The model under review builds one solid part; all positions refer to its coordinate system, in mm. A direction names the side the tool comes from. Give positions to 0.01 mm unless a question says otherwise; leave off trailing zeros. Order: outer loops, then holes, each group sorted by start corner. A loop starts at its lowest first (then second) coordinate and runs counter-clockwise, first axis right, second up.
```python
from build123d import *

# Parameters (mm, degrees)
F1_DEPTH = 19.05
F2_R     = 28.575
F3_DEPTH = 19.051
F4_R     = 12.7
F5_DEPTH = 15.24


with BuildPart() as f1:
    # F0 (on Top) → F1 (new body)
    with BuildSketch(Plane.XY):
        with BuildLine():
            ThreePointArc((133.35, 127), (125.910512, 144.960512), (107.95, 152.4))
            Line((107.95, 152.4), (0, 152.4))
            Line((0, 152.4), (0, -152.4))
            Line((0, -152.4), (107.95, -152.4))
            ThreePointArc((107.95, -152.4), (125.910512, -144.960512), (133.35, -127))
            Line((133.35, -127), (133.35, 127))
        make_face()
        with BuildLine():
            Line((0, -152.4), (0, 152.4))
            Line((0, 152.4), (-107.95, 152.4))
            ThreePointArc((-107.95, 152.4), (-125.910512, 144.960512), (-133.35, 127))
            Line((-133.35, 127), (-133.35, -127))
            ThreePointArc((-133.35, -127), (-125.910512, -144.960512), (-107.95, -152.4))
            Line((-107.95, -152.4), (0, -152.4))
        make_face()
    extrude(amount=F1_DEPTH)

    # F2 (on face) → F3 (cut, through all)
    with BuildSketch(Plane.XY.offset(19.05)):
        with Locations((-55.88, 100.965)):
            Circle(F2_R)
        with Locations((-55.88, 33.655)):
            Circle(F2_R)
        with Locations((-55.88, -33.655)):
            Circle(F2_R)
        with Locations((-55.88, -100.965)):
            Circle(F2_R)
        with Locations((55.88, -100.965)):
            Circle(F2_R)
        with Locations((55.88, -33.655)):
            Circle(F2_R)
        with Locations((55.88, 33.655)):
            Circle(F2_R)
        with Locations((55.88, 100.965)):
            Circle(F2_R)
    extrude(amount=-F3_DEPTH, mode=Mode.SUBTRACT)

    # F4 (on face) → F5 (cut)
    with BuildSketch(Plane.XY.offset(19.05)):
        with Locations((0, 96.52)):
            Circle(F4_R)
        with Locations((0, -96.52)):
            Circle(F4_R)
    extrude(amount=-F5_DEPTH, mode=Mode.SUBTRACT)


solid = f1.part
```
Item 1: Take a section at B-B (y = -96.52). Give the boundary of the cut face in (x, z), and give its area (3 significant figures).
Values found:
outline: (-133.35, 0) - (-84.11, 0) - (-84.11, 19.05) - (-133.35, 19.05) - close; (-27.65, 0) - (27.65, 0) - (27.65, 19.05) - (12.7, 19.05) - (12.7, 3.81) - (-12.7, 3.81) - (-12.7, 19.05) - (-27.65, 19.05) - close; (84.11, 0) - (133.35, 0) - (133.35, 19.05) - (84.11, 19.05) - close
area: 2,540 mm2
Item 2: Draft analysis for pull direction X (two halves, no side actions). For faces 1 (the flat face through (-2, 2, 19.05)), 2 (the cylindrical face through (125.71, -145.16, 9.39)), 3 (the cylindrical face through (-62.07, 73.07, 9.66)), state which applies: released by +X, released by -X, zero draft, split by the parting line, or undercut.
Values found:
face 1: zero draft
face 2: released by +X
face 3: undercut
Item 3: Clearance check with a flat-ended pin moving along its axis: pin 1 Ø7.5 at (x, y) = (6, 96) entering from +Z. State where the tip first meets the part, or that it passes through.
Values found:
pin 1: stops at z = 3.81
Item 4: Take a section at C-C (z = 7.5). Give the number of separate pieces and of enclosed holes in the cut face, and give its area (3 significant figures).
Values found:
separate pieces: 1
enclosed holes: 10
area: 59,200 mm2
Item 5: For faces 4 (the flat face through (0, -96, 3.81)), 5 (the cylindrical face through (-126.11, -144.76, 9.39)), list the 3-axis set-ups (+Z, -Z, +X, -X, +Y, -Y) from which the entire face can be reached by the end or side of a thin tool; tool diameter is ignored.
Values found:
face 4: +Z
face 5: +Z, -Z, -X, -Y
Item 6: For line 1 (X direction, y = -33, z = 3.75); line 2 (Y direction, x = -55.88, z = 5.25); line 3 (Y direction, x = 58, z = 11.5), list the stretches that pass through material, from the lowest coordinate up.
Values found:
line 1: x = -133.35 to -84.45, -27.31 to 27.31, 84.45 to 133.35
line 2: y = -152.4 to -129.54, -72.39 to -62.23, -5.08 to 5.08, 62.23 to 72.39, 129.54 to 152.4
line 3: y = -152.4 to -129.46, -72.47 to -62.15, -5.16 to 5.16, 62.15 to 72.47, 129.46 to 152.4
Item 7: Take a section at D-D (x = 0). Give the boundary of the cut face in (y, z).
Values found:
outline: (-152.4, 0) - (152.4, 0) - (152.4, 19.05) - (109.22, 19.05) - (109.22, 3.81) - (83.82, 3.81) - (83.82, 19.05) - (-83.82, 19.05) - (-83.82, 3.81) - (-109.22, 3.81) - (-109.22, 19.05) - (-152.4, 19.05) - close
Item 8: Take a section at A-A (x = 55.88). Give the boundary of the cut face in (y, z).
Values found:
outline: (-152.4, 0) - (-129.54, 0) - (-129.54, 19.05) - (-152.4, 19.05) - close; (-72.39, 0) - (-62.23, 0) - (-62.23, 19.05) - (-72.39, 19.05) - close; (-5.08, 0) - (5.08, 0) - (5.08, 19.05) - (-5.08, 19.05) - close; (62.23, 0) - (72.39, 0) - (72.39, 19.05) - (62.23, 19.05) - close; (129.54, 0) - (152.4, 0) - (152.4, 19.05) - (129.54, 19.05) - close
